Part model, mm, in its own coordinate system. Round coordinates to 2 decimals unless told otherwise and drop trailing zeros. Loops run counter-clockwise (first coordinate to the right, second up) from the corner with the lowest first, then second, coordinate; pieces in that order, holes last.
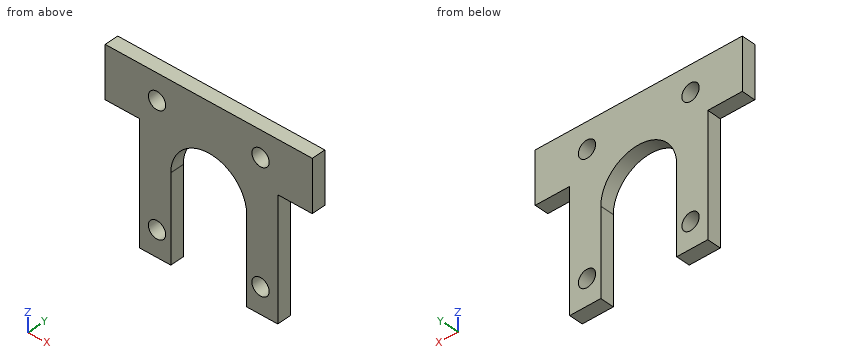
from build123d import *

# Parameters (mm, degrees)
F0_R     = 2.5
F1_DEPTH = 4


with BuildPart() as f1:
    # F0 (on Front) → F1 (new body)
    with BuildSketch(Plane.XZ):
        with BuildLine():
            ThreePointArc((-11, 0), (0, 11), (11, 0))
            Line((11, 0), (11, -25))
            Line((11, -25), (20, -25))
            Line((20, -25), (20, 10))
            Line((20, 10), (30, 10))
            Line((30, 10), (30, 25))
            Line((30, 25), (-30, 25))
            Line((-30, 25), (-30, 10))
            Line((-30, 10), (-20, 10))
            Line((-20, 10), (-20, -25))
            Line((-20, -25), (-11, -25))
            Line((-11, -25), (-11, 0))
        make_face()
        with Locations((-15, -17.5)):
            Circle(F0_R, mode=Mode.SUBTRACT)
        with Locations((15, -17.5)):
            Circle(F0_R, mode=Mode.SUBTRACT)
        with Locations((-15, 17.5)):
            Circle(F0_R, mode=Mode.SUBTRACT)
        with Locations((15, 17.5)):
            Circle(F0_R, mode=Mode.SUBTRACT)
    extrude(amount=F1_DEPTH)


solid = f1.part
1) Slice it at C-C, the plane y = -2.4. Give the cut face in (x, z).
Values:
outline: (-30, 10) - (-20, 10) - (-20, -25) - (-11, -25) - (-11, 0) arc R11 cw to (11, 0) - (11, -25) - (20, -25) - (20, 10) - (30, 10) - (30, 25) - (-30, 25) - close; hole circle Ø5 at (-15, -17.5); hole circle Ø5 at (-15, 17.5); hole circle Ø5 at (15, -17.5); hole circle Ø5 at (15, 17.5)
2) Slice it at D-D, the plane z = 17.5. Give the cut face in (x, y), then the cut area to 3 significant figures.
Values:
outline: (-30, -4) - (-17.5, -4) - (-17.5, 0) - (-30, 0) - close; (-12.5, -4) - (12.5, -4) - (12.5, 0) - (-12.5, 0) - close; (17.5, -4) - (30, -4) - (30, 0) - (17.5, 0) - close
area: 200 mm2
3) Wall check: line 1 along Z through (x, y) = (-15, -2.7); line 2 along X through (y, z) = (-3.35, -10); line 3 along Z through (x, y) = (13, -0.9). Give the ranges that are in metal, low to high.
Values:
line 1: z = -25 to -20, -15 to 15, 20 to 25
line 2: x = -20 to -11, 11 to 20
line 3: z = -25 to -19, -16 to 16, 19 to 25
4) Slice it at B-B, the plane z = -2.5. Give the cut face in (x, y).
Values:
outline: (-20, -4) - (-11, -4) - (-11, 0) - (-20, 0) - close; (11, -4) - (20, -4) - (20, 0) - (11, 0) - close
5) Slice it at A-A, the plane x = 16.5. Give the cut face in (y, z).
Values:
outline: (-4, -25) - (0, -25) - (0, -19.5) - (-4, -19.5) - close; (-4, -15.5) - (0, -15.5) - (0, 15.5) - (-4, 15.5) - close; (-4, 19.5) - (0, 19.5) - (0, 25) - (-4, 25) - close
6) Drop flat-ended pins along their axis: pin 1 Ø2 at (y, z) = (-2, -10) entering from +X; pin 2 Ø2 at (x, y) = (23, -3) entering from -Z; pin 3 Ø2 at (y, z) = (-2.5, -6.5) entering from -X. Give the stop position or say it passes through.
Values:
pin 1: stops at x = 20
pin 2: stops at z = 10
pin 3: stops at x = -20
